Verification items for the finished model (mm, model axes). A direction names the side the tool comes from. Coordinates: 2 decimals unless noted, no trailing zeros. Write each loop counter-clockwise with the first axis right and the second up, starting at its lowest first coordinate (ties: lowest second). Pieces come first, ordered by that corner, then holes.
```python
from build123d import *

# Parameters (mm, degrees)
F0_W     = 80.01
F0_H     = 80.01
F1_DEPTH = 12.7
F2_W     = 74.93
F2_H     = 74.93
F3_DEPTH = 10.16
F4_R     = 12.7
F5_DEPTH = 25.4


with BuildPart() as f1:
    # F0 (on Front) → F1 (new body)
    with BuildSketch(Plane.XZ):
        Rectangle(F0_W, F0_H)
    extrude(amount=F1_DEPTH)

    # F2 (on face) → F3 (cut)
    with BuildSketch(Plane(origin=(0, 0, 0), x_dir=(-1, 0, 0), z_dir=(0, 1, 0))):
        Rectangle(F2_W, F2_H)
    extrude(amount=-F3_DEPTH, mode=Mode.SUBTRACT)

    # F4 (on face) → F5 (cut)
    with BuildSketch(Plane(origin=(0, -10.16, 0), x_dir=(-1, 0, 0), z_dir=(0, 1, 0))):
        with Locations((19.145673, 18.554756)):
            Circle(F4_R)
    extrude(amount=-F5_DEPTH, mode=Mode.SUBTRACT)


solid = f1.part
```
1. Material ranges on L1, parallel to X at y = -5.5, z = 4 (3 decimals); L2, parallel to Y at x = -8, z = -30, recorded low to high.
2. Sectioned sample at D-D, the plane x = 8. Record the boundary of the cut face in (y, z) (3 decimals).
3. Gauge pin test, flat ends, axial feed: P1, Ø6, axis at x = 12, z = -13.5, coming from the +Y side; P2, Ø23, axis at x = -19.15, z = 18.55, coming from the -Y side. Record the tip position at first contact, or that the pin passes through.
4. Sectioned sample at C-C, the plane z = 4.5. Record the boundary of the cut face in (x, y) (3 decimals), and give its area (3 significant figures).
5. Sectioned sample at A-A, the plane y = -4.25. Record the boundary of the cut face in (x, z) (3 decimals), and give its area (3 significant figures).
6. Draft check along Z on faces 1 (the flat face through (-40.005, -6, -1)), 2 (the flat face through (-1, -6, 40.005)), 3 (the flat face through (-37.465, -5, -1)). Enter one of: pulls with the +Z half, pulls with the -Z half, needs draft (parallel to the pull), parting line crosses it, or undercut.
7. Tool access check on faces 4 (the cylindrical face through (-16.393, -11.412, 6.157)), 5 (the flat face through (37.465, -5, -1)). Record the directions out of +Z, -Z, +X, -X, +Y, -Y that give a thin tool (end or side, any length) a straight path to the whole face; none if there is none.
8. Sectioned sample at B-B, the plane x = -11.5. Record the boundary of the cut face in (y, z) (3 decimals).
Outcome:
1. L1: x = -40.005 to -37.465, 37.465 to 40.005
1. L2: y = -12.7 to -10.16
2. outline: (-12.7, -40.005) - (0, -40.005) - (0, -37.465) - (-10.16, -37.465) - (-10.16, 37.465) - (0, 37.465) - (0, 40.005) - (-12.7, 40.005) - close
3. P1: stops at y = -10.16
3. P2: passes through
4. outline: (-40.005, -12.7) - (40.005, -12.7) - (40.005, 0) - (37.465, 0) - (37.465, -10.16) - (-37.465, -10.16) - (-37.465, 0) - (-40.005, 0) - close
4. area: 255 mm2
5. outline: (-40.005, -40.005) - (40.005, -40.005) - (40.005, 40.005) - (-40.005, 40.005) - close; hole (-37.465, -37.465) - (37.465, -37.465) - (37.465, 37.465) - (-37.465, 37.465) - close
5. area: 787 mm2
6. face 1: needs draft
6. face 2: pulls with the +Z half
6. face 3: undercut
7. face 4: +Y, -Y
7. face 5: +Y
8. outline: (-12.7, -40.005) - (0, -40.005) - (0, -37.465) - (-10.16, -37.465) - (-10.16, 8.414) - (-12.7, 8.414) - close; (-12.7, 28.695) - (-10.16, 28.695) - (-10.16, 37.465) - (0, 37.465) - (0, 40.005) - (-12.7, 40.005) - close
